```python
from build123d import *

# Parameters (mm, degrees)
SKETCH1_R           = 21
SKETCH1_R_2         = 5
BOSS_EXTRUDE1_DEPTH = 10
FILLET1_R           = 50
FILLET2_R           = 70
BOSS_EXTRUDE2_START = -15
SKETCH2_R           = 23.5
SKETCH2_R_2         = 21
BOSS_EXTRUDE2_DEPTH = 15


with BuildPart() as part:
    # Sketch1 → Boss-Extrude1 (new body)
    with BuildSketch(Plane.XY):
        with BuildLine():
            Line((-54.365348895, 227.889389357), (-99.36593713, 245.389389357))
            Line((-99.36593713, 245.389389357), (-144.365348895, 227.889389357))
            ThreePointArc((-144.365348895, 227.889389357), (-156.865348895, 215.389389357), (-144.365348895, 202.889389357))
            Line((-144.365348895, 202.889389357), (-99.36593713, 185.389389357))
            Line((-99.36593713, 185.389389357), (-54.365348895, 202.889389357))
            ThreePointArc((-54.365348895, 202.889389357), (-41.865348895, 215.389389357), (-54.365348895, 227.889389357))
        make_face()
        with Locations((-99.36593713, 215.389389357)):
            Circle(SKETCH1_R, mode=Mode.SUBTRACT)
        with Locations((-54.365348895, 215.389389357)):
            Circle(SKETCH1_R_2, mode=Mode.SUBTRACT)
        with Locations((-144.365348895, 215.389389357)):
            Circle(SKETCH1_R_2, mode=Mode.SUBTRACT)
    extrude(amount=BOSS_EXTRUDE1_DEPTH)

    # Fillet1
    fillet1_edges = [part.edges().sort_by_distance(p)[0] for p in [
        (-99.36593713, 185.389389357, 5),
        (-99.36593713, 245.389389357, 5),
    ]]
    fillet(fillet1_edges, radius=FILLET1_R)

    # Fillet2
    fillet2_edges = [part.edges().sort_by_distance(p)[0] for p in [
        (-54.365348895, 202.889389357, 5),
        (-144.365348895, 202.889389357, 5),
        (-144.365348895, 227.889389357, 5),
        (-54.365348895, 227.889389357, 5),
    ]]
    fillet(fillet2_edges, radius=FILLET2_R)

    # Sketch2 → Boss-Extrude2 (add)
    with BuildSketch(Plane.XY.offset(10).offset(BOSS_EXTRUDE2_START)):
        with Locations((-99.36593713, 215.389389357)):
            Circle(SKETCH2_R)
        with Locations((-99.36593713, 215.389389357)):
            Circle(SKETCH2_R_2, mode=Mode.SUBTRACT)
    extrude(amount=BOSS_EXTRUDE2_DEPTH)


solid = part.part
```
For this review, take the finished solid that the model builds, in its own axes (mm). A direction names the side the tool comes from. Round coordinates to 2 decimals unless told otherwise and drop trailing zeros. Loops run counter-clockwise (first coordinate to the right, second up) from the corner with the lowest first, then second, coordinate; pieces in that order, holes last.
Q1. Mouldability with a two-part tool opening along Y and no side actions: class faces 1 (the face through (-127.674, 196.398, 4.93)), 2 (the face through (-117, 203, -5)), 3 (the face through (-55.45, 210.51, 4.93)) as +Y half, -Y half, draft (parallel to the pull), parting line (faces both ways), or undercut.
Result sheet:
face 1: -Y half
face 2: draft
face 3: undercut
Q2. Add section B-B on x = -106. Write out the cut boundary in (y, z).
Result sheet:
outline: (189.48, 0) - (192.85, 0) - (192.85, -5) - (195.46, -5) - (195.46, 10) - (189.48, 10) - close; (235.31, -5) - (237.93, -5) - (237.93, 0) - (241.3, 0) - (241.3, 10) - (235.31, 10) - close
Q3. Insertion check: pin 1 Ø2 at (x, z) = (-91, 6.5) entering from -Y; pin 2 Ø16 at (x, y) = (-54.37, 215.39) entering from -Z; pin 3 Ø2 at (x, z) = (-138, 3) entering from +Y; pin 4 Ø6 at (x, y) = (-144.37, 215.39) entering from +Z. Each pin has a flat end and moves straight along its axis. Give the tip position at first contact, or say it passes through.
Result sheet:
pin 1: stops at y = 189.58
pin 2: stops at z = 0
pin 3: stops at y = 230.75
pin 4: passes through
Q4. Add section D-D on y = 224. Write out the cut boundary in (x, z), plus the area to 3 significant figures.
Result sheet:
outline: (-153.43, 0) - (-121.23, 0) - (-121.23, -5) - (-118.52, -5) - (-118.52, 10) - (-153.43, 10) - close; (-80.21, -5) - (-77.5, -5) - (-77.5, 0) - (-45.3, 0) - (-45.3, 10) - (-80.21, 10) - close
area: 725 mm2
Q5. Machinability: for faces 4 (the face through (-127.39, 234.49, 4.93)), 5 (the face through (-102.43, 238.69, -2.54)), which of the approach directions +Z, -Z, +X, -X, +Y, -Y give a long, thin tool a straight path to every point of the face, cutting with its end or side? Answer none if there is none.
Result sheet:
face 4: +Z, -Z, -X, +Y
face 5: -Z
Q6. Add section A-A on y = 212. Write out the cut boundary in (x, z), plus the area to 3 significant figures.
Result sheet:
outline: (-156.4, 0) - (-148.04, 0) - (-148.04, 10) - (-156.4, 10) - close; (-140.69, 0) - (-122.62, 0) - (-122.62, -5) - (-120.09, -5) - (-120.09, 10) - (-140.69, 10) - close; (-78.64, -5) - (-76.11, -5) - (-76.11, 0) - (-58.04, 0) - (-58.04, 10) - (-78.64, 10) - close; (-50.69, 0) - (-42.33, 0) - (-42.33, 10) - (-50.69, 10) - close
area: 604 mm2
Q7. To check wall thickness, follow line 1 along X through (y, z) = (217.5, 7); line 2 along Z through (x, y) = (-67.5, 231.5); line 3 along X through (y, z) = (223, -3). State the ranges of each line that lie inside material, in increasing order.
Result sheet:
line 1: x = -156.69 to -148.9, -139.83 to -120.26, -78.47 to -58.9, -49.83 to -42.04
line 2: z = 0 to 10
line 3: x = -121.6 to -118.94, -79.79 to -77.13
Q8. Add section C-C on z = 5. Write out the cut boundary in (x, y).
Result sheet:
outline: (-147.18, 203.21) arc R70 cw to (-137.58, 200.25) - (-117.49, 192.44) arc R50 ccw to (-81.24, 192.44) - (-61.15, 200.25) arc R70 cw to (-51.55, 203.21) arc R12.5 ccw to (-51.55, 227.57) arc R70 cw to (-61.15, 230.53) - (-81.24, 238.34) arc R50 ccw to (-117.49, 238.34) - (-137.58, 230.53) arc R70 cw to (-147.18, 227.57) arc R12.5 ccw to start; hole circle Ø10 at (-144.37, 215.39); hole circle Ø42 at (-99.37, 215.39); hole circle Ø10 at (-54.37, 215.39)
